Work out the finished part from the listing and answer in its coordinate system (mm). Give positions to 0.01 mm unless a question says otherwise; leave off trailing zeros. Loops run counter-clockwise (first coordinate to the right, second up) from the corner with the lowest first, then second, coordinate; pieces in that order, holes last. Notation, with made-up numbers: M -19,43.25 L 4,43.25 A34 cw 4,74.25 Z; hole C 62.25,-21.75 d4. An arc over 180 degrees is marked long. Use a Markdown table: item, result.
```python
from build123d import *

# Parameters (mm, degrees)
SKETCH1_W                    = 38.1
SKETCH1_H                    = 1.5875
F_36_0_1065_DIAMETER_HOLE1_D = 2.7051
CIRPATTERN1_COUNT            = 12


with BuildPart() as part:
    # Sketch1 → Revolve1 (revolve)
    with BuildSketch(Plane.XY):
        with Locations((-28.575, 0.79375)):
            Rectangle(SKETCH1_W, SKETCH1_H)
    revolve(axis=Axis((0, 55, 0), (0, -1, 0)))

    # #36 (0.1065) Diameter Hole1 (through all)
    with Locations(Plane(origin=(0, 1.5875, 0), x_dir=(1, 0, 0), z_dir=(0, 1, 0))):
        with Locations((-42.8625, 0)):
            f_36_0_1065_diameter_hole1 = Hole(F_36_0_1065_DIAMETER_HOLE1_D / 2)

    # CirPattern1: #36 (0.1065) Diameter Hole1 ×12 about axis
    cirpattern1_axis = Axis((0, 0, 0), (0, 1, 0))
    for i in range(1, CIRPATTERN1_COUNT):
        add(f_36_0_1065_diameter_hole1.rotate(cirpattern1_axis, i * 360 / CIRPATTERN1_COUNT), mode=Mode.SUBTRACT)


solid = part.part
```
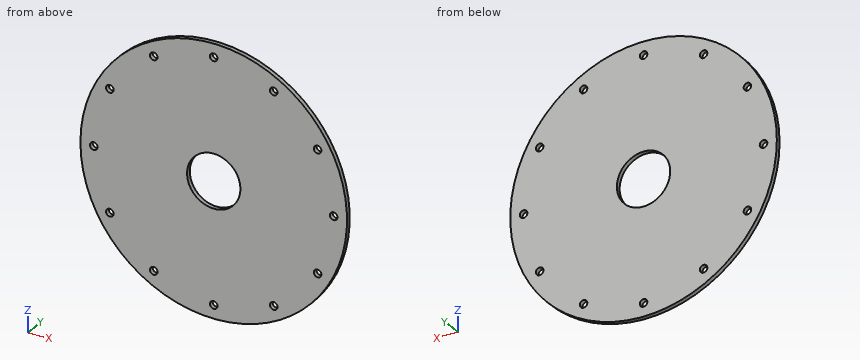
(1) Given P1, Ø4.5, axis at x = -37.12, z = 21.43, coming from the +Y side; P2, Ø1.6, axis at x = -21.43, z = -37.12, coming from the -Y side, each flat-ended and moving along its own axis, determine where each tip first touches the part or whether it passes through.
Entries:
| item | result |
|---|---|
| P1 | stops at y = 1.59 |
| P2 | passes through |
(2) A cutting plane is placed at A-A (x = 0). Write down the section's boundary in (y, z) (1 decimal).
Entries:
| item | result |
|---|---|
| outline | M 0,-47.6 L 1.6,-47.6 L 1.6,-44.2 L 0,-44.2 Z; M 0,-41.5 L 1.6,-41.5 L 1.6,-9.5 L 0,-9.5 Z; M 0,9.5 L 1.6,9.5 L 1.6,41.5 L 0,41.5 Z; M 0,44.2 L 1.6,44.2 L 1.6,47.6 L 0,47.6 Z |
(3) A cutting plane is placed at C-C (z = 16.5). Write down the section's boundary in (x, y).
Entries:
| item | result |
|---|---|
| outline | M -44.68,0 L 44.68,0 L 44.68,1.59 L -44.68,1.59 Z |
(4) Consider probe 1 along Z at (x, y) = (-37.5, 1); probe 2 along X at (y, z) = (0.4, 36); probe 3 along Z at (x, y) = (36.5, 0.25). Determine where each line is inside the solid, lowest interval first. Write a range as [from, to].
Entries:
| item | result |
|---|---|
| probe 1 | z = [-29.36, -22.73], [-20.13, 20.13], [22.73, 29.36] |
| probe 2 | x = [-31.18, -22.19], [-20.67, 20.67], [22.19, 31.18] |
| probe 3 | z = [-30.59, -22.63], [-20.23, 20.23], [22.63, 30.59] |
(5) A cutting plane is placed at B-B (z = 0). Write down the section's boundary in (x, y) (1 decimal), and give its area (3 significant figures).
Entries:
| item | result |
|---|---|
| outline | M -47.6,0 L -44.2,0 L -44.2,1.6 L -47.6,1.6 Z; M -41.5,0 L -9.5,0 L -9.5,1.6 L -41.5,1.6 Z; M 9.5,0 L 41.5,0 L 41.5,1.6 L 9.5,1.6 Z; M 44.2,0 L 47.6,0 L 47.6,1.6 L 44.2,1.6 Z |
| area | 112 mm² |
(6) A cutting plane is placed at D-D (x = -16). Write down the section's boundary in (y, z).
Entries:
| item | result |
|---|---|
| outline | M 0,-44.86 L 1.59,-44.86 L 1.59,44.86 L 0,44.86 Z |
